Build history of the part. All positions in model axes, mm. A direction names the side the tool comes from. Coordinates: 2 decimals unless noted, no trailing zeros. Order: outer loops, then holes, each group sorted by start corner. A loop starts at its lowest first (then second) coordinate and runs counter-clockwise, first axis right, second up. Notation, with made-up numbers: (31.25, 78.25) - (77.25, 78.25) arc R36 ccw to (77.25, 115.25) - close; hole circle Ø8 at (16, -37). An arc over 180 degrees is marked (long way). One line per item, written item: value.
from build123d import *

# Parameters (mm, degrees)
SKETCH_2_R          = 15
EXTRUDE_1_DEPTH     = 19
SKETCH_3_R          = 10
CUT_EXTRUDE_1_DEPTH = 25


with BuildPart() as part:
    # 스케치1 → 회전1 (revolve)
    with BuildSketch(Plane.XY):
        with BuildLine():
            Line((0, 0), (0, 17.5))
            Line((0, 17.5), (5, 17.5))
            ThreePointArc((5, 17.5), (27.465304528, 15.62548151), (50, 15))
            Line((50, 15), (67, 15))
            Line((67, 15), (67, 17.5))
            Line((67, 17.5), (72, 17.5))
            Line((72, 17.5), (72, 15))
            Line((72, 15), (75, 15))
            Line((75, 15), (75, 10))
            Line((75, 10), (60, 10))
            Line((60, 10), (60, 0))
            Line((60, 0), (0, 0))
        make_face()
    revolve(axis=Axis((0, 0, 0), (1, 0, 0)))

    # 스케치2 → 보스-돌출1 (add)
    with BuildSketch(Plane.XY):
        with Locations((17.5, 0)):
            Circle(SKETCH_2_R)
    extrude(amount=EXTRUDE_1_DEPTH)

    # 스케치3 → 컷-돌출1 (cut)
    with BuildSketch(Plane.XY.offset(19)):
        with Locations((17.5, 0)):
            Circle(SKETCH_3_R)
    extrude(amount=-CUT_EXTRUDE_1_DEPTH, mode=Mode.SUBTRACT)


solid = part.part
1. Probe line 1 along X through (y, z) = (0.5, 16); line 2 along Z through (x, y) = (66, 0); line 3 along X through (y, z) = (4, 16.5). List the from-to ranges inside material, lowest first.
Values found:
line 1: x = 0 to 7.51, 27.49 to 32.49, 67 to 72
line 2: z = -15 to -10, 10 to 15
line 3: x = 0 to 8.33, 26.67 to 31.96, 67 to 72
2. Band-saw the part on D-D, the plane x = 17.5. Give the cut face in (y, z).
Values found:
outline: (-15, 6.38) arc R16.3 ccw (long way) to (15, 6.38) - (15, 19) - (10, 19) - (10, -6) - (-10, -6) - (-10, 19) - (-15, 19) - close
3. Band-saw the part on A-A, the plane z = 0. Give the cut face in (x, y).
Values found:
outline: (0, -17.5) - (5, -17.5) arc R406.25 cw to (50, -15) - (67, -15) - (67, -17.5) - (72, -17.5) - (72, -15) - (75, -15) - (75, -10) - (60, -10) - (60, 10) - (75, 10) - (75, 15) - (72, 15) - (72, 17.5) - (67, 17.5) - (67, 15) - (50, 15) arc R406.25 cw to (5, 17.5) - (0, 17.5) - close; hole circle Ø20 at (17.5, 0)
4. Band-saw the part on B-B, the plane x = 69. Give the cut face in (y, z), and give its area (3 significant figures).
Values found:
outline: circle Ø35 at (0, 0); hole circle Ø20 at (0, 0)
area: 648 mm2
5. Band-saw the part on C-C, the plane y = 0. Give the cut face in (x, z).
Values found:
outline: (0, -17.5) - (5, -17.5) arc R406.25 cw to (50, -15) - (67, -15) - (67, -17.5) - (72, -17.5) - (72, -15) - (75, -15) - (75, -10) - (60, -10) - (60, 10) - (75, 10) - (75, 15) - (72, 15) - (72, 17.5) - (67, 17.5) - (67, 15) - (50, 15) arc R406.25 cw to (32.5, 15.38) - (32.5, 19) - (27.5, 19) - (27.5, -6) - (7.5, -6) - (7.5, 19) - (2.5, 19) - (2.5, 17.5) - (0, 17.5) - close
6. 3-axis set-ups, long thin cutter, end or side, ignore diameter. For faces 4 (the face through (0, 0, 0)), 5 (the face through (17, 0, -6)), 6 (the face through (73.521, -14.985, 0.66)), 7 (the face through (67, -13, 8)), 8 (the face through (2.535, -3.794, -17.084)): which of +Z, -Z, +X, -X, +Y, -Y reach the whole face in a straight line?
Values found:
face 4: +Z, -Z, -X, +Y, -Y
face 5: +Z
face 6: +X
face 7: none
face 8: -X
7. Two-plate mould, pull along Z, no slides. Class faces 1 (the face through (27.3, -3.1, 19)), 2 (the face through (72, 13, 8)), 3 (the face through (60, 0, 0)): pulls with the +Z half, pulls with the -Z half, needs draft (parallel to the pull), parting line crosses it, or undercut.
Values found:
face 1: pulls with the +Z half
face 2: needs draft
face 3: undercut
8. Flat gauge pins, fed straight in: P1, Ø2, axis at x = 11.5, z = -9.5, coming from the -Y side; P2, Ø1.5, axis at x = 56, y = 1.5, coming from the -Z side; P3, Ø12, axis at x = 17.5, y = 0, coming from the +Z side; P4, Ø8, axis at y = 3, z = -4, coming from the -X side. Where does each tip first touch, or does it go through?
Values found:
P1: stops at y = -14.53
P2: stops at z = -14.98
P3: stops at z = -6
P4: stops at x = 0
